Geometry: final body of the model. Coordinates: model frame, mm. A direction names the side the tool comes from. Coordinates: 2 decimals unless noted, no trailing zeros. Order: outer loops, then holes, each group sorted by start corner. A loop starts at its lowest first (then second) coordinate and runs counter-clockwise, first axis right, second up. Notation, with made-up numbers: (-31.5, -36) -> (-5.5, -36) arc R26 ccw to (-5.5, -3) -> close; hole circle Ø3 at (75.25, 69.5). An arc over 180 degrees is marked (long way). Answer in a Markdown table with one row per item. Add a question column.
1) Section query D-D on z = -34. Return the cut outline in (x, y), then the cut area to 3 significant figures.
2) Ray query, line 1 (Y direction, x = -5.75, z = 0); line 2 (Y direction, x = -40.5, z = -27); line 3 (Z direction, x = -3.5, y = 264). Return the intervals inside material, ascending. Write a range as from..to.
3) Set-up query: faces 1 (the face through (-12, 305, 0)), 2 (the face through (-13, 13, -15)), 3 (the face through (0, 12.2, 3.5)). Return all of +Z, -Z, +X, -X, +Y, -Y with unobstructed straight access to the full face (end or side cutting, diameter ignored); none if empty.
4) Section query B-B on y = 9. Return the cut outline in (x, z).
5) Pull-direction query (Y, two-part tool) for faces 4 (the face through (-0.012, 169.425, -0.55)), 5 (the face through (-12, 13, 15)), 6 (the face through (-12, -15, 0)); classes: +Y half, -Y half, draft (parallel to the pull), parting line (faces both ways), or undercut.
6) Section query A-A on y = 256. Return the cut outline in (x, z), then the cut area to 3 significant figures.
7) Contact query for flat-ended pins moving along their axis: P1, Ø9, axis at y = 3, z = 5.5, coming from the -X side; P2, Ø20, axis at x = -7.5, y = 11, coming from the -Z side; P3, Ø5, axis at x = -1, y = 246, coming from the +Z side; P4, Ø7, axis at x = -11.5, z = -4, coming from the -Y side. Output: stop coordinate, or through.
8) Section query C-C on x = 24.5. Return the cut outline in (y, z), then the cut area to 3 significant figures.
```python
from build123d import *

# Parameters (mm, degrees)
SKETCH1_R           = 15
SKETCH1_R_2         = 12.5
BOSS_EXTRUDE1_DEPTH = 25
CUT_EXTRUDE1_DEPTH  = 280
FILLET1_R           = 5
FILLET2_R           = 5
SKETCH3_R           = 11.5
CUT_EXTRUDE2_DEPTH  = 300
SKETCH4_R           = 42
BOSS_EXTRUDE2_DEPTH = 2


with BuildPart() as part:
    # Sketch1 → Boss-Extrude1 (new body)
    # profile 1 of 2: a face of its own
    with BuildSketch(Plane(origin=(0, 0, 0), x_dir=(0, 0, -1), z_dir=(1, 0, 0))):
        with BuildLine():
            ThreePointArc((-15, 0), (0, 15), (15, 0))
            Line((15, 0), (15, 305))
            Line((15, 305), (-15, 305))
            Line((-15, 305), (-15, 0))
        make_face()
    # profile 2 of 2: a face of its own
    with BuildSketch(Plane(origin=(0, 0, 0), x_dir=(0, 0, -1), z_dir=(1, 0, 0))):
        Circle(SKETCH1_R)
        Circle(SKETCH1_R_2, mode=Mode.SUBTRACT)
    extrude(amount=-BOSS_EXTRUDE1_DEPTH)

    # Sketch2 → Cut-Extrude1 (cut)
    with BuildSketch(Plane(origin=(0, 305, 0), x_dir=(1, 0, 0), z_dir=(0, 1, 0))):
        with BuildLine():
            Line((0, -15), (0, 0))
            ThreePointArc((0, 0), (-12.5, -12.5), (-25, 0))
            Line((-25, 0), (-25, -15))
            Line((-25, -15), (0, -15))
        make_face()
        with BuildLine():
            ThreePointArc((-25, 0), (-12.5, 12.5), (0, 0))
            Line((0, 0), (0, 15))
            Line((0, 15), (-25, 15))
            Line((-25, 15), (-25, 0))
        make_face()
    extrude(amount=-CUT_EXTRUDE1_DEPTH, mode=Mode.SUBTRACT)

    # Fillet1
    # the kernel refuses this fillet: 5 mm, written as the material it adds along each edge
    with BuildSketch(Plane(origin=(-12.5, 25, 0), x_dir=(1, 0, 0), z_dir=(0, 0, -1))) as fillet1_piece_1_section:
        with BuildLine():
            CenterArc((12.5 + FILLET1_R, -FILLET1_R), FILLET1_R, 90, 90)
            Line((12.5, -FILLET1_R), (12.5, 0))
            Line((12.5, 0), (12.5 + FILLET1_R, 0))
        make_face()
    fillet1_piece_1 = revolve(axis=Axis((-12.5, 25, 0), (0, -1, 0)), revolution_arc=180, mode=Mode.PRIVATE)
    fillet1_piece_1 = split(fillet1_piece_1, bisect_by=Plane(origin=(-12.5, 26.425263387, 15), z_dir=(0, 0, -1)), keep=Keep.TOP, mode=Mode.PRIVATE)
    fillet1_piece_1 = split(fillet1_piece_1, bisect_by=Plane(origin=(-25, 26.425263387, 13.925263387), z_dir=(1, 0, 0)), keep=Keep.TOP, mode=Mode.PRIVATE)
    fillet1_piece_1 = split(fillet1_piece_1, bisect_by=Plane(origin=(0, 26.425263387, 13.925263387), z_dir=(-1, 0, 0)), keep=Keep.TOP, mode=Mode.PRIVATE)
    add(fillet1_piece_1)

    # Fillet2
    # the kernel refuses this fillet: 5 mm, written as the material it adds along each edge
    with BuildSketch(Plane(origin=(-12.5, 25, 0), x_dir=(-0.5389483633149527, 0, 0.8423388045674577), z_dir=(0.8423388045674577, 0, 0.5389483633149527))) as fillet2_piece_1_section:
        with BuildLine():
            CenterArc((12.5 + FILLET2_R, -FILLET2_R), FILLET2_R, 90, 90)
            Line((12.5 + FILLET2_R, 0), (12.5, 0))
            Line((12.5, 0), (12.5, -FILLET2_R))
        make_face()
    fillet2_piece_1 = revolve(axis=Axis((-12.5, 25, 0), (0, -1, 0)), revolution_arc=294.775843921, mode=Mode.PRIVATE)
    fillet2_piece_1 = split(fillet2_piece_1, bisect_by=Plane(origin=(-25, 27.5000003, -12.555440979), z_dir=(1, 0, 0)), keep=Keep.TOP, mode=Mode.PRIVATE)
    fillet2_piece_1 = split(fillet2_piece_1, bisect_by=Plane(origin=(0, 27.5000003, -12.555440979), z_dir=(-1, 0, 0)), keep=Keep.TOP, mode=Mode.PRIVATE)
    fillet2_piece_1 = split(fillet2_piece_1, bisect_by=Plane(origin=(-12.5, 27.5000003, -15), z_dir=(0, 0, 1)), keep=Keep.TOP, mode=Mode.PRIVATE)
    add(fillet2_piece_1)

    # Sketch3 → Cut-Extrude2 (cut)
    with BuildSketch(Plane(origin=(0, 305, 0), x_dir=(1, 0, 0), z_dir=(0, 1, 0))):
        with Locations(Location((-12.5, 0, 0), (0, 0, 270))):
            Circle(SKETCH3_R)
    extrude(amount=-CUT_EXTRUDE2_DEPTH, mode=Mode.SUBTRACT)

    # Sketch4 → Boss-Extrude2 (add)
    with BuildSketch(Plane(origin=(0, 305, 0), x_dir=(1, 0, 0), z_dir=(0, 1, 0))):
        with Locations(Location((-12.5, 0, 0), (0, 0, 270))):
            Circle(SKETCH4_R)
    extrude(amount=BOSS_EXTRUDE2_DEPTH)


solid = part.part
```
Result:
| question | item | result |
|---|---|---|
| 1 | outline | (-37.16, 305) -> (12.16, 305) -> (12.16, 307) -> (-37.16, 307) -> close |
| 1 | area | 98.6 mm2 |
| 2 | line 1 | -15..-12.5, 305..307 |
| 2 | line 2 | 305..307 |
| 2 | line 3 | -8.67..-7.16, 7.16..8.67 |
| 3 | face 1 | none |
| 3 | face 2 | -Z, +X, -X, -Y |
| 3 | face 3 | +Z, -Z, +X, -Y |
| 4 | outline | (-25, -15) -> (0, -15) -> (0, -8.67) -> (-4.95, -8.67) arc R11.5 cw to (-20.05, -8.67) -> (-25, -8.67) -> close; (-25, 8.67) -> (-20.05, 8.67) arc R11.5 cw to (-4.95, 8.67) -> (0, 8.67) -> (0, 15) -> (-25, 15) -> close |
| 5 | face 4 | undercut |
| 5 | face 5 | draft |
| 5 | face 6 | -Y half |
| 6 | outline | circle Ø25 at (-12.5, 0); hole circle Ø23 at (-12.5, 0) |
| 6 | area | 75.4 mm2 |
| 7 | P1 | through |
| 7 | P2 | z = -15 |
| 7 | P3 | z = 8.67 |
| 7 | P4 | y = -14.99 |
| 8 | outline | (305, -19.87) -> (307, -19.87) -> (307, 19.87) -> (305, 19.87) -> close |
| 8 | area | 79.5 mm2 |
